Part print with two shaded views. Sizes in mm from the minimum x, y, z corner. A direction names the side the tool comes from. Round coordinates to 2 decimals unless told otherwise and drop trailing zeros. Order: outer loops, then holes, each group sorted by start corner. A loop starts at its lowest first (then second) coordinate and runs counter-clockwise, first axis right, second up. Notation, with made-up numbers: M -28,47.5 L -17,47.5 A29 cw -17,67.5 Z; hole C 58.25,-21 d3. An arc over 180 degrees is marked long. Return JSON: item names as keys, results as strings. Group by question number.
Item 1: Which spindle directions (+Z, -Z, +X, -X, +Y, -Y) get a long thin tool onto all of the face, cutting with end or side? Do the marked faces 4 and 5. Say none if no direction does.
Item 2: Pin check, flat tips, straight feed: pin 1 Ø4 at (x, z) = (20, 7.5) entering from +Y; pin 2 Ø2 at (y, z) = (9, 3.5) entering from -X. Stop position of each tip, or through.
Item 3: Slice it at A-A on x = 10. Write the cut outline in (y, z), then the cut area to 3 significant figures.
Item 4: Pull direction X, two halves, no side cores. Call the marked faces 1, 2 and 3: pulls with the +X half, pulls with the -X half, needs draft (parallel to the pull), parting line crosses it, or undercut.
Item 5: Slice it at D-D on y = 7.5. Write the cut outline in (x, z), then the cut area to 3 significant figures.
Item 6: Slice it at B-B on z = 7.5. Write the cut outline in (x, y), then the cut area to 3 significant figures.
Item 7: Probe line 1 along X through (y, z) = (1.25, 7.5); line 2 along Z through (x, y) = (10, 1.4); line 3 along Y through (x, z) = (19.5, 2.25). List the from-to ranges inside material, lowest first.
Item 8: Slice it at C-C on z = 13.25. Write the cut outline in (x, y), then the cut area to 3 significant figures.
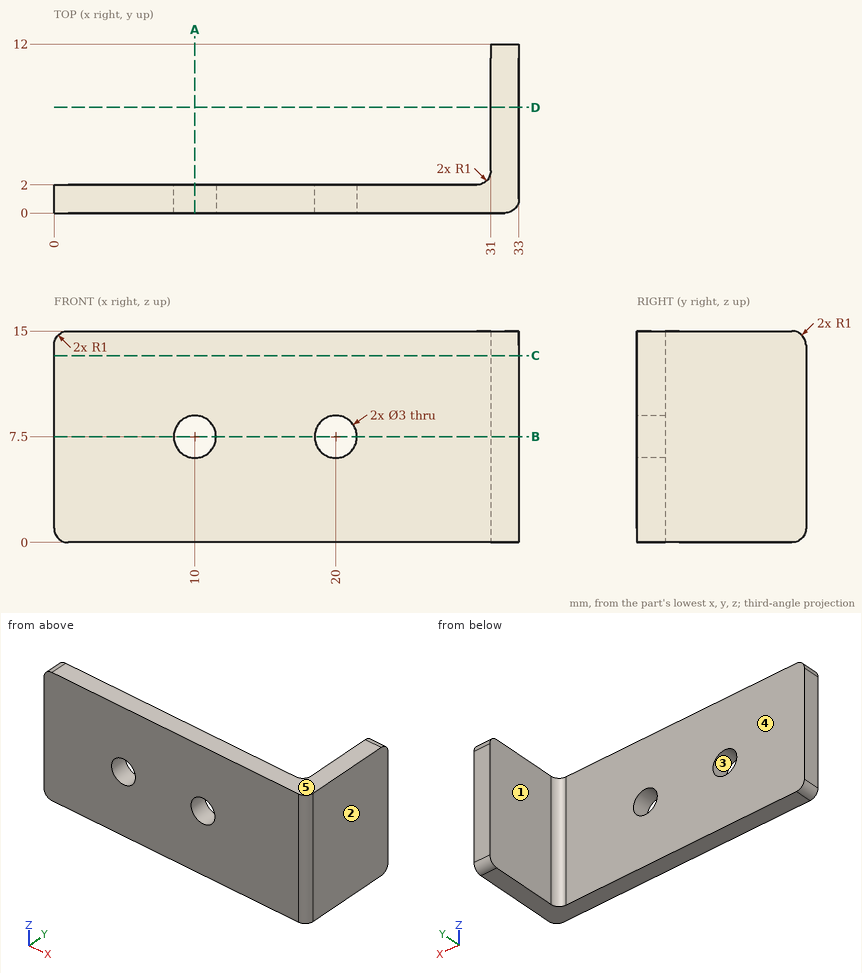
Output values:
{
 "1": {"face 4": "+Z, -Z, -X, +Y", "face 5": "+Z, +X, -X, +Y, -Y"},
 "2": {"pin 1": "y = 2", "pin 2": "x = 31"},
 "3": {"outline": "M 0,0 L 2,0 L 2,6 L 0,6 Z; M 0,9 L 2,9 L 2,15 L 0,15 Z", "area": "24.0 mm²"},
 "4": {"face 1": "pulls with the -X half", "face 2": "pulls with the +X half", "face 3": "undercut"},
 "5": {"outline": "M 31,0 L 33,0 L 33,15 L 31,15 Z", "area": "30.0 mm²"},
 "6": {"outline": "M 0,0 L 8.5,0 L 8.5,2 L 0,2 Z; M 11.5,0 L 18.5,0 L 18.5,2 L 11.5,2 Z; M 21.5,0 L 32,0 A1 ccw 33,1 L 33,12 L 31,12 L 31,3 A1 cw 30,2 L 21.5,2 Z", "area": "74.0 mm²"},
 "7": {"line 1": "0 to 8.5, 11.5 to 18.5, 21.5 to 33", "line 2": "0 to 6, 9 to 15", "line 3": "0 to 2"},
 "8": {"outline": "M 0,0 L 32,0 A1 ccw 33,1 L 33,12 L 31,12 L 31,3 A1 cw 30,2 L 0,2 Z", "area": "86.0 mm²"}
}
